The listing builds one solid part. Answer for the finished solid, in the listing's coordinates (mm). Face numbers are marked on the shaded views. A direction names the side the tool comes from. Give positions to 0.01 mm unless a question says otherwise; leave off trailing zeros. Write each loop counter-clockwise with the first axis right and the second up, starting at its lowest first coordinate (ties: lowest second). Pieces come first, ordered by that corner, then holes. Notation, with made-up numbers: (65.5, -13.75) -> (70.5, -13.75) arc R20 cw to (70.5, -6.75) -> close; hole circle Ø2 at (15.25, 77). An arc over 180 degrees is marked (long way). Use CSV: the item, a comma, the result in double quotes. Start each with the question number.
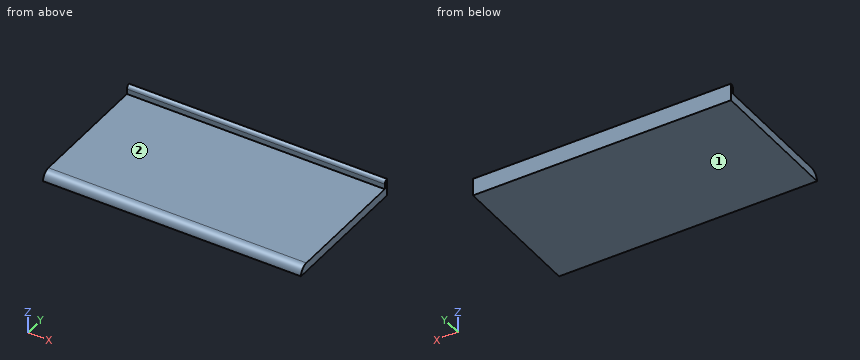
Autodesk Inventor part; units mm, degrees
ref_plane "YZ Plane" through (0, 0, 0) normal (1, 0, 0) x (0, 1, 0)
ref_plane "XZ Plane" through (0, 0, 0) normal (0, 1, 0) x (-1, 0, 0)
ref_plane "XY Plane" through (0, 0, 0) normal (0, 0, 1) x (1, 0, 0)
sketch "Sketch1" plane through (0, 0, 0) normal (0, 0, 1) x (1, 0, 0)
  line L0 (0, 0) -> (1483.3333, 0)
  line L1 (1483.3333, 0) -> (1483.3333, 790)
  line L2 (1483.3333, 790) -> (0, 790)
  line L3 (0, 790) -> (0, 0)
  dimension "ancho" = 1483.3333
  dimension "d1" = 790
extrude "Extrusion1" add sketch "Sketch1" along normal blind 50
fillet "Fillet1" radius 50 1 edges at (741.6667, 0, 50)
sketch "Sketch2" plane through (1483.3333, 790, 50) normal (1, 0, 0) x (0, 0, -1)
  line L0 (50, 0) -> (-50, 0)
  line L1 (-50, 0) -> (-50, 0)
  line L2 (-30, -20) -> (50, -20)
  line L3 (50, -20) -> (50, 0)
  arc A0 (-50, 0) -> (-30, -20) centre (-30, 0) ccw
  point P0 (50, -790)
  point P1 (-50, -20)
  dimension "d5" = 100
  dimension "d6" = 20
  dimension "d7" = 20
extrude "Extrusion2" add sketch "Sketch2" against normal up to surface (1483.3333 mm away)
properties part number "meson"
Q1. Section B-B on y = 173.5 is taken. Give the vertices of the cut face in (x, z), then the cut area to 3 significant figures.
Q2. For the marked faces 1 and 2, determine the directions among +Z, -Z, +X, -X, +Y, -Y from which every point of the face is accessible in a straight line to the end or side of a thin tool.
Q3. Straight lines are drawn through the part: L1, parallel to Z at x = 194, y = 566.5; L2, parallel to Y at x = 379.5, z = 55; L3, parallel to Y at x = 1363, z = 14. For each, find the intervals that lie inside material, in ascending order.
Q4. Flat-ended cylindrical pins translate along their axes: pin 1 Ø10 at (x, z) = (744, 86.5) entering from -Y; pin 2 Ø3 at (x, y) = (495.5, 169.5) entering from +Z; pin 3 Ø24 at (x, z) = (885.5, 62.5) entering from -Y. Find the tip coordinate at first contact, or state that the pin passes through.
Output:
1,outline,"(0, 0) -> (1483.33, 0) -> (1483.33, 50) -> (0, 50) -> close"
1,area,"74,200 mm²"
2,face 1,"-Z, +X, -X, +Y, -Y"
2,face 2,"+Z, +X, -X, -Y"
3,L1,"0 to 50"
3,L2,"770 to 790"
3,L3,"2 to 790"
4,pin 1,"y = 770.06"
4,pin 2,"z = 50"
4,pin 3,"y = 770"
